Source: CAD feature listing. Evaluate the final solid. Frame: model axes, mm. A direction names the side the tool comes from. Coordinates: 2 decimals unless noted, no trailing zeros. Write each loop counter-clockwise with the first axis right and the second up, starting at its lowest first coordinate (ties: lowest second). Pieces come first, ordered by that corner, then holes. Notation, with made-up numbers: (-22, 75.25) -> (0, 75.25) arc R24 cw to (0, 102.25) -> close; hole circle Ø3 at (73.25, 8). An arc over 180 degrees is marked (long way). One line per item, written item: value. Start each with the question number.
1. Section query A-A, the plane x = 88.9. Output: boundary loops of the cut face in (y, z) (3 decimals), and give its area (3 significant figures).
2. First-contact query: P1, Ø3.5, axis at x = -9.5, z = 0, coming from the +Y side; P2, Ø4, axis at x = 51.5, y = 6.5, coming from the -Z side; P3, Ø16, axis at x = 88.9, z = 0, coming from the +Y side. Flat tips, straight axial feed; report the tip coordinate or a pass-through.
3. Access query for faces 4 (the flat face through (76.2, 9, 0)), 5 (the cylindrical face through (100.15, 5.26, -13.08)), 6 (the cylindrical face through (-81.404, 7.577, 4.779)). Directions: +Z, -Z, +X, -X, +Y, -Y. A direction counts if a zero-diameter tool reaches every point of the face in a straight line with its end or side. Return the directions, or none.
4. Section query C-C, the plane x = 52. Output: boundary loops of the cut face in (y, z) (3 decimals).
5. Section query B-B, the plane y = 9. Output: boundary loops of the cut face in (x, z) (3 decimals).
6. Line query: line 1 (X direction, y = 2.2, z = 0) (3 decimals); line 2 (X direction, y = 9, z = -3.25); line 3 (Z direction, x = 9.5, y = 3.05) (3 decimals). Output: solid intervals per line, ascending.
7. Mould query, pull axis Z, two halves, no side actions, for faces 1 (the cylindrical face through (-84.997, 2.254, 0.513)), 2 (the flat face through (-101.6, 5, 0)), 3 (the flat face through (1, 3, -14.605)). Classes: released by +Z, released by -Z, zero draft, split by the parting line, or undercut.
from build123d import *

# Parameters (mm, degrees)
SKETCH1_R                = 13.97
SKETCH1_R_2              = 1.275
BOSS_EXTRUDE1_DEPTH      = 3.048
BOSS_EXTRUDE2_DEPTH      = 7.62
BOSS_EXTRUDE2_DEPTH_BACK = 3.048
SKETCH2_R                = 8.89
SKETCH2_R_2              = 1.275
CUT_EXTRUDE2_DEPTH       = 107.252483849
SKETCH6_R                = 8.89
SKETCH6_R_2              = 3.937
BOSS_EXTRUDE3_DEPTH      = 4.572
FILLET2_R                = 3.048


with BuildPart() as part:
    # Sketch1 → Boss-Extrude1 (new body)
    with BuildSketch(Plane(origin=(0, 0, 0), x_dir=(1, 0, 0), z_dir=(0, 1, 0))):
        with Locations(Location((0, 0, 0), (0, 0, 90))):
            Circle(SKETCH1_R)
        with Locations(Location((0, 9.5, 0), (0, 0, 90))):
            Circle(SKETCH1_R_2, mode=Mode.SUBTRACT)
        with Locations(Location((9.5, 0, 0), (0, 0, 90))):
            Circle(SKETCH1_R_2, mode=Mode.SUBTRACT)
        with Locations(Location((0, -9.5, 0), (0, 0, 90))):
            Circle(SKETCH1_R_2, mode=Mode.SUBTRACT)
        with Locations(Location((-9.5, 0, 0), (0, 0, 90))):
            Circle(SKETCH1_R_2, mode=Mode.SUBTRACT)
    extrude(amount=BOSS_EXTRUDE1_DEPTH)

    # Sketch2 → Boss-Extrude2 (add, two sides: drawn at the far end of the back side and taken through both)
    with BuildSketch(Plane(origin=(0, 3.048, 0), x_dir=(1, 0, 0), z_dir=(0, 1, 0)).offset(-BOSS_EXTRUDE2_DEPTH_BACK)):
        with BuildLine():
            Line((-96.52, -14.605), (96.52, -14.605))
            ThreePointArc((96.52, -14.605), (100.112102448, -13.117102448), (101.6, -9.525))
            Line((101.6, -9.525), (101.6, 9.525))
            ThreePointArc((101.6, 9.525), (100.112102448, 13.117102448), (96.52, 14.605))
            Line((96.52, 14.605), (-96.52, 14.605))
            ThreePointArc((-96.52, 14.605), (-100.112102448, 13.117102448), (-101.6, 9.525))
            Line((-101.6, 9.525), (-101.6, -9.525))
            ThreePointArc((-101.6, -9.525), (-100.112102448, -13.117102448), (-96.52, -14.605))
        make_face()
        with Locations(Location((-88.9, 0, 0), (0, 0, 270))):
            Circle(SKETCH2_R, mode=Mode.SUBTRACT)
        with Locations(Location((88.9, 0, 0), (0, 0, 270))):
            Circle(SKETCH2_R, mode=Mode.SUBTRACT)
        with Locations(Location((9.5, 0, 0), (0, 0, 90))):
            Circle(SKETCH2_R_2, mode=Mode.SUBTRACT)
        with Locations(Location((0, 9.5, 0), (0, 0, 90))):
            Circle(SKETCH2_R_2, mode=Mode.SUBTRACT)
        with Locations(Location((-9.5, 0, 0), (0, 0, 90))):
            Circle(SKETCH2_R_2, mode=Mode.SUBTRACT)
        with Locations(Location((0, -9.5, 0), (0, 0, 90))):
            Circle(SKETCH2_R_2, mode=Mode.SUBTRACT)
    extrude(amount=BOSS_EXTRUDE2_DEPTH + BOSS_EXTRUDE2_DEPTH_BACK)

    # Sketch5 → Cut-Extrude2 (cut, through all)
    with BuildSketch(Plane(origin=(0, 0, -14.605), x_dir=(-1, 0, 0), z_dir=(0, 0, -1))):
        Polygon((-76.2, 3.81), (0, 3.81), (76.2, 3.81), (76.2, 10.668), (-76.2, 10.668), align=None)
    extrude(amount=-CUT_EXTRUDE2_DEPTH, mode=Mode.SUBTRACT)

    # Sketch6 → Boss-Extrude3 (add)
    # profile 1 of 2: a face of its own
    with BuildSketch(Plane.XZ):
        with Locations(Location((-88.9, 0, 0), (0, 0, 90))):
            Circle(SKETCH6_R)
        with Locations(Location((-88.9, 0, 0), (0, 0, 270))):
            Circle(SKETCH6_R_2, mode=Mode.SUBTRACT)
    # profile 2 of 2: a face of its own
    with BuildSketch(Plane.XZ):
        with Locations(Location((88.9, 0, 0), (0, 0, 90))):
            Circle(SKETCH6_R)
        with Locations(Location((88.9, 0, 0), (0, 0, 270))):
            Circle(SKETCH6_R_2, mode=Mode.SUBTRACT)
    extrude(amount=-BOSS_EXTRUDE3_DEPTH)

    # Fillet2
    fillet2_edges = [part.edges().sort_by_distance(p)[0] for p in [
        (-76.2, 3.81, 0),
        (76.2, 3.81, 0),
    ]]
    fillet(fillet2_edges, radius=FILLET2_R)


solid = part.part
Computed values:
1. outline: (0, -14.605) -> (10.668, -14.605) -> (10.668, -8.89) -> (4.572, -8.89) -> (4.572, -3.937) -> (0, -3.937) -> close; (0, 3.937) -> (4.572, 3.937) -> (4.572, 8.89) -> (10.668, 8.89) -> (10.668, 14.605) -> (0, 14.605) -> close
1. area: 167 mm²
2. P1: stops at y = 3.81
2. P2: passes through
2. P3: stops at y = 4.57
3. face 4: +Z, -Z, +Y
3. face 5: -Z, +X, +Y, -Y
3. face 6: +Y
4. outline: (0, -14.605) -> (3.81, -14.605) -> (3.81, 14.605) -> (0, 14.605) -> close
5. outline: (-101.6, -9.525) arc R5.08 ccw to (-96.52, -14.605) -> (-76.2, -14.605) -> (-76.2, 14.605) -> (-96.52, 14.605) arc R5.08 ccw to (-101.6, 9.525) -> close; (76.2, -14.605) -> (96.52, -14.605) arc R5.08 ccw to (101.6, -9.525) -> (101.6, 9.525) arc R5.08 ccw to (96.52, 14.605) -> (76.2, 14.605) -> close; hole circle Ø17.78 at (-88.9, 0); hole circle Ø17.78 at (88.9, 0)
6. line 1: x = -101.6 to -92.837, -84.963 to -10.775, -8.225 to 8.225, 10.775 to 84.963, 92.837 to 101.6
6. line 2: x = -101.6 to -97.17, -80.63 to -76.2, 76.2 to 80.63, 97.17 to 101.6
6. line 3: z = -14.605 to -1.275, 1.275 to 14.605
7. face 1: undercut
7. face 2: zero draft
7. face 3: released by -Z
